Autodesk Inventor part; units mm, degrees
ref_plane "YZ Plane" through (0, 0, 0) normal (1, 0, 0) x (0, 1, 0)
ref_plane "XZ Plane" through (0, 0, 0) normal (0, 1, 0) x (-1, 0, 0)
ref_plane "XY Plane" through (0, 0, 0) normal (0, 0, 1) x (1, 0, 0)
sketch "Skizze1" plane through (0, 0, 0) normal (0, 1, 0) x (-1, 0, 0)
  line L0 (10, 50) -> (-10, 50)
  line L1 (-10, 50) -> (-10, -50)
  line L2 (-10, -50) -> (10, -50)
  line L3 (10, -50) -> (10, 50)
  line L4 (10, 50) -> (-10, -50) construction
  line L5 (-10, 50) -> (10, -50) construction
  point P0 (0, 0)
  dimension "d0" = 100
  dimension "d1" = 20
extrude "Extrusion1" add sketch "Skizze1" along normal mid plane 20
sketch "Skizze2" plane through (0, 10, 0) normal (0, 1, 0) x (1, 0, 0)
  line L0 (-10, 50) -> (-10, -50)
  line L1 (-10, 0) -> (10, 0)
  line L2 (10, -50) -> (10, 50)
  point P0 (0, 0)
  point P1 (0, -30)
  point P2 (0, 30)
  dimension "d4" = 60
hole "Bohrung1" at (0, 10, 30) at (0, 10, -30) direction (0, -1, 0) diameter 10.106 depth 12 tip angle 118
sketch "Skizze3" plane through (0, 10, 0) normal (0, 1, 0) x (1, 0, 0)
  circle A0 centre (0, -30) radius 5.053
  point P0 (0, 0)
hole "Bohrung2" at (0, 10, 30) direction (0, -1, 0) diameter 4.134 end through all
sketch "Skizze4" plane through (0, 10, 0) normal (0, 1, 0) x (1, 0, 0)
  circle A0 centre (0, 30) radius 5.053
  point P0 (0, 0)
hole "Bohrung3" at (0, 10, -30) direction (0, -1, 0) diameter 4.134 end through all
sketch "Skizze5" plane through (0, 10, 0) normal (0, 1, 0) x (1, 0, 0)
  line L0 (-10, -50) -> (-10, 50)
  line L1 (-10, 0) -> (10, 0)
  line L2 (10, 50) -> (10, -50)
  point P0 (0, 0)
  point P1 (0, -42.5)
  point P2 (0, 0)
  point P3 (0, 42.5)
  point P4 (0, 0)
  dimension "d26" = 85
hole "Bohrung4" at (0, 10, 0) at (0, 10, -42.5) at (0, 10, 42.5) direction (0, -1, 0) diameter 4.5 depth 20 counterbore diameter 8 counterbore depth 4.4
properties part number "106.014.01_Anbindung_Vereinzelung" material "Aluminium 6061"
Here's how the part is built. I have some questions about the finished solid (model axes, mm). A direction names the side the tool comes from. Round coordinates to 2 decimals unless told otherwise and drop trailing zeros. Write each loop counter-clockwise with the first axis right and the second up, starting at its lowest first coordinate (ties: lowest second). Pieces come first, ordered by that corner, then holes.
1. If we mould it in two halves opening along X, with no side actions, what happens to faces 3 (the flat face through (2, 5.6, 44)), 4 (the flat face through (0, 0, 50)), 5 (the conical face through (-0.863, -3.682, -27.918)), 6 (the flat face through (-10, 0, -1))? For each: released by +X, released by -X, zero draft, split by the parting line, or undercut.
2. I need wall thicknesses on L1, parallel to Z at x = 0, y = 7.3; L2, parallel to Z at x = 0, y = -4.75; L3, parallel to X at y = -6.25, z = 0. Which ranges of each line are inside material? Lowest first, please.
3. Will these pins go through, and if not, where does the flat tip stop? pin 1 Ø7 at (x, z) = (0, 0) entering from +Y; pin 2 Ø6 at (x, z) = (0, 30) entering from +Y.
4. Suppose I cut it at C-C (x = 0). State how many separate pieces and enclosed holes the cut face has, and give its area (3 significant figures).
5. Suppose I cut it at A-A (z = 42.5). List the corners of the cut face in (x, y) for me, and give its area (3 significant figures).
6. Suppose I cut it at D-D (y = 7.5). List the corners of the cut face in (x, z) for me, and give its area (3 significant figures).
7. Suppose I cut it at B-B (y = -1). List the corners of the cut face in (x, z) for me.
8. For faces 1 (the cylindrical face through (2.4, 7.8, 39.3)), 2 (the cylindrical face through (-0.62, -6.94, 31.97)), which set-ups out of +Z, -Z, +X, -X, +Y, -Y let a thin tool reach every point of the face, with its end or its side?
Answer sheet:
1. face 3: undercut
1. face 4: zero draft
1. face 5: undercut
1. face 6: released by -X
2. L1: z = -50 to -46.5, -38.5 to -35.05, -24.95 to -4, 4 to 24.95, 35.05 to 38.5, 46.5 to 50
2. L2: z = -50 to -44.75, -40.25 to -32.07, -27.93 to -2.25, 2.25 to 27.93, 32.07 to 40.25, 44.75 to 50
2. L3: x = -10 to -2.25, 2.25 to 10
3. pin 1: stops at y = 5.6
3. pin 2: stops at y = -3.23
4. separate pieces: 6
4. enclosed holes: 0
4. area: 1,360 mm2
5. outline: (-10, -10) - (-2.25, -10) - (-2.25, 5.6) - (-4, 5.6) - (-4, 10) - (-10, 10) - close; (2.25, -10) - (10, -10) - (10, 10) - (4, 10) - (4, 5.6) - (2.25, 5.6) - close
5. area: 295 mm2
6. outline: (-10, -50) - (10, -50) - (10, 50) - (-10, 50) - close; hole circle Ø10.11 at (0, -30); hole circle Ø10.11 at (0, 30); hole circle Ø8 at (0, -42.5); hole circle Ø8 at (0, 0); hole circle Ø8 at (0, 42.5)
6. area: 1,690 mm2
7. outline: (-10, -50) - (10, -50) - (10, 50) - (-10, 50) - close; hole circle Ø10.11 at (0, -30); hole circle Ø10.11 at (0, 30); hole circle Ø4.5 at (0, -42.5); hole circle Ø4.5 at (0, 0); hole circle Ø4.5 at (0, 42.5)
8. face 1: +Y
8. face 2: +Y, -Y
